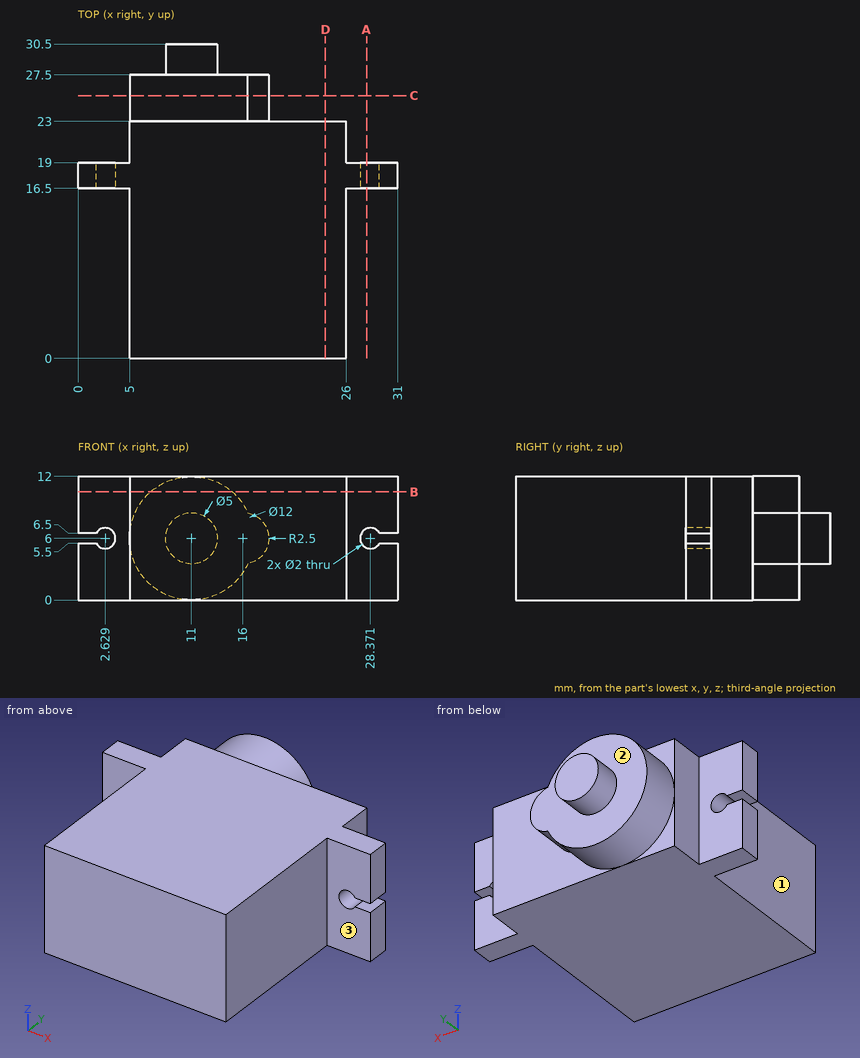
Here's the drawing with two shaded views (mm, measured from the low corner). I have some questions. A direction names the side the tool comes from. Coordinates: 2 decimals unless noted, no trailing zeros. Loops run counter-clockwise (first coordinate to the right, second up) from the corner with the lowest first, then second, coordinate; pieces in that order, holes last. Notation, with made-up numbers: (22.25, -14.5) -> (69.25, -14.5) arc R30 ccw to (69.25, 18.5) -> close; hole circle Ø5 at (33.25, 46). An arc over 180 degrees is marked (long way). Answer as a JSON object with one key per item and string values.
1) For P1, Ø4, axis at x = 29, z = 5.5, coming from the +Y side; P2, Ø1.5, axis at y = 24, z = 9.5, coming from the +X side; P3, Ø6, axis at x = 26.5, z = 1.5, coming from the +Y side, each with a flat end and sliding along its axis, tell me the tip position at first contact or that it passes through.
Results:
{"P1": "stops at y = 19", "P2": "stops at x = 16.33", "P3": "stops at y = 23"}
2) Imagine slicing it at C-C (y = 25.5). Please give me the cut outline in (x, z) (1 decimal).
Results:
{"outline": "(16.5, 3.5) arc R2.5 ccw to (16.5, 8.5) arc R6 ccw (long way) to start"}
3) Imagine slicing it at A-A (x = 28). Please give me the cut outline in (y, z).
Results:
{"outline": "(16.5, 0) -> (19, 0) -> (19, 5.07) -> (16.5, 5.07) -> close; (16.5, 6.93) -> (19, 6.93) -> (19, 12) -> (16.5, 12) -> close"}
4) Imagine slicing it at B-B (z = 10.5). Please give me the cut outline in (x, y).
Results:
{"outline": "(0, 16.5) -> (5, 16.5) -> (5, 0) -> (26, 0) -> (26, 16.5) -> (31, 16.5) -> (31, 19) -> (26, 19) -> (26, 23) -> (14.97, 23) -> (14.97, 27.5) -> (7.03, 27.5) -> (7.03, 23) -> (5, 23) -> (5, 19) -> (0, 19) -> close"}
5) For the marked faces 1, 2 and 3, which set-ups out of +Z, -Z, +X, -X, +Y, -Y let a thin tool reach every point of the face, with its end or its side?
Results:
{"face 1": "+Z, -Z, -X, -Y", "face 2": "+Y", "face 3": "+Z, -Z, +X, -Y"}
6) If I drill on line 1 (Y direction, x = 29.5, z = 4.25); line 2 (X direction, y = 2.5, z = 3); line 3 (Y direction, x = 10.5, z = 2.5), over which ranges is the centre line in solid material (lowest first)?
Results:
{"line 1": "y = 16.5 to 19", "line 2": "x = 5 to 26", "line 3": "y = 0 to 27.5"}
7) Imagine slicing it at D-D (x = 24). Please give me the cut outline in (y, z).
Results:
{"outline": "(0, 0) -> (23, 0) -> (23, 12) -> (0, 12) -> close"}
